Could you check a few things on this drawing? It's one solid part, dimensions in mm from its lowest x, y, z. A direction names the side the tool comes from. Give positions to 0.01 mm unless a question says otherwise; leave off trailing zeros. Order: outer loops, then holes, each group sorted by start corner. A loop starts at its lowest first (then second) coordinate and runs counter-clockwise, first axis right, second up.
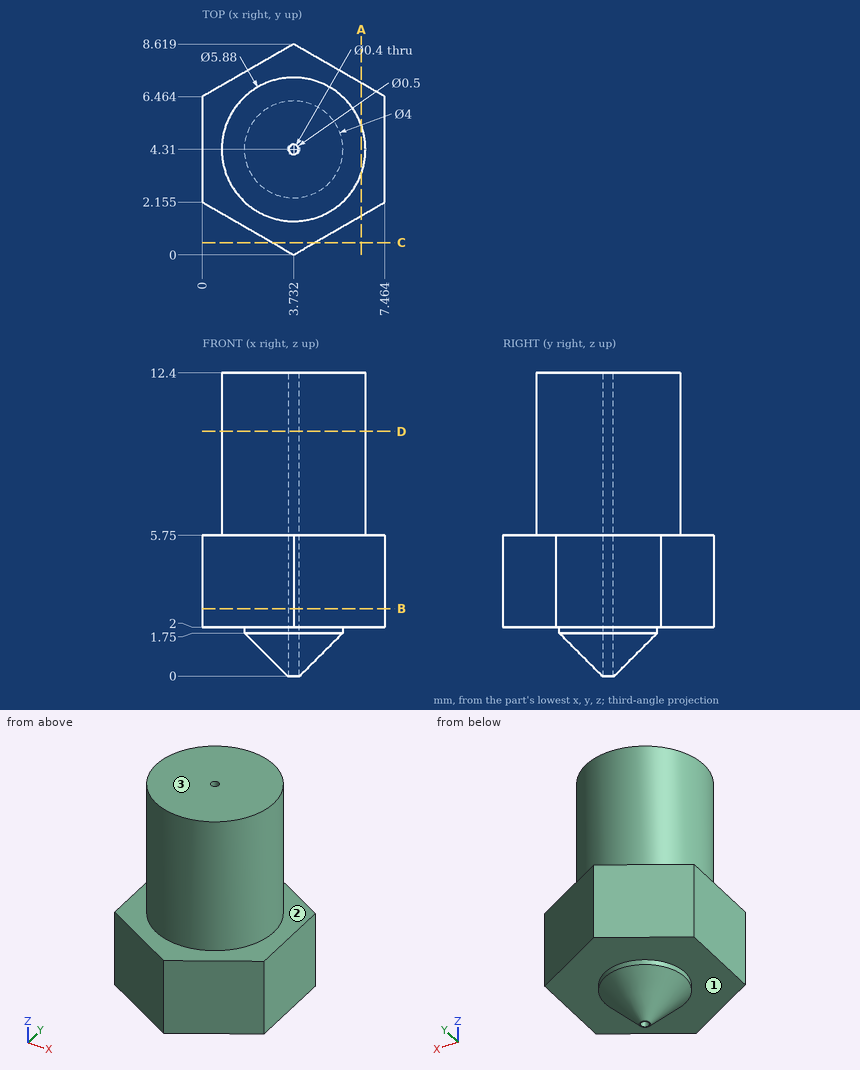
Q1. For the marked faces 1, 2 and 3, which set-ups out of +Z, -Z, +X, -X, +Y, -Y let a thin tool reach every point of the face, with its end or its side?
Filled sheet:
face 1: -Z
face 2: +Z
face 3: +Z, +X, -X, +Y, -Y
Q2. If we section it at B-B on z = 2.75: List the corners of the cut face in (x, y) for me (1 decimal).
Filled sheet:
outline: (0, 2.2) - (3.7, 0) - (7.5, 2.2) - (7.5, 6.5) - (3.7, 8.6) - (0, 6.5) - close; hole circle Ø0.4 at (3.7, 4.3)
Q3. If we section it at D-D on z = 10: List the corners of the cut face in (x, y) for me.
Filled sheet:
outline: circle Ø5.88 at (3.73, 4.31); hole circle Ø0.4 at (3.73, 4.31)
Q4. I'm going to push flat-ended pins straight in: P1, Ø2, axis at x = 4.5, z = 6.5, coming from the -Y side; P2, Ø4, axis at x = 1.5, z = 4.5, coming from the +Y side (1 decimal). Where does each tip first touch, or does it pass through?
Filled sheet:
P1: stops at y = 0.06
P2: stops at y = 8.5
Q5. I need wall thicknesses on L1, parallel to Z at x = 1, y = 3.75; L2, parallel to Z at x = 4.25, y = 8; L3, parallel to X at y = 1.75, z = 7.75 (1 decimal). Which ranges of each line are inside material? Lowest first, please.
Filled sheet:
L1: z = 2 to 12.4
L2: z = 2 to 5.75
L3: x = 2.3 to 5.2
Q6. If we section it at C-C on y = 0.5: List the corners of the cut face in (x, z) for me.
Filled sheet:
outline: (2.87, 2) - (4.6, 2) - (4.6, 5.75) - (2.87, 5.75) - close
Q7. If we section it at A-A on x = 6.5: List the corners of the cut face in (y, z) for me.
Filled sheet:
outline: (1.6, 2) - (7.02, 2) - (7.02, 5.75) - (5.3, 5.75) - (5.3, 12.4) - (3.32, 12.4) - (3.32, 5.75) - (1.6, 5.75) - close
